The model under review builds one solid part; all positions refer to its coordinate system, in mm. A direction names the side the tool comes from. Coordinates: 2 decimals unless noted, no trailing zeros. Order: outer loops, then holes, each group sorted by start corner. A loop starts at its lowest first (then second) coordinate and runs counter-clockwise, first axis right, second up.
```python
from build123d import *

# Parameters (mm, degrees)
SKETCH1_W                    = 444
SKETCH1_H                    = 24
BASE_FLANGE1_DEPTH           = 1.214
EDGE_FLANGE1_STRIP_W         = 7.284
EDGE_FLANGE1_STRIP_H         = 1.214
EDGE_FLANGE1_STRIP_CUT_DEPTH = 444
EDGE_FLANGE1_DEPTH           = 444
SKETCH9_R                    = 2.5
CUT_EXTRUDE1_DEPTH           = 10


# Sheet-metal steps are written as plain solids
with BuildPart() as part:
    # Sketch1 → Base-Flange1 (new body)
    with BuildSketch(Plane(origin=(0, 0, 0), x_dir=(1, 0, 0), z_dir=(0, 1, 0))):
        Rectangle(SKETCH1_W, SKETCH1_H)
    extrude(amount=BASE_FLANGE1_DEPTH)

    # Edge-Flange1 strip (across the edge) → Edge-Flange1 strip cut (cut)
    with BuildSketch(Plane(origin=(-222, 1.214, 12), x_dir=(0, 0, -1), z_dir=(1, 0, 0))):
        with Locations((-1.214, -0.607)):
            Rectangle(EDGE_FLANGE1_STRIP_W, EDGE_FLANGE1_STRIP_H)
    extrude(amount=EDGE_FLANGE1_STRIP_CUT_DEPTH, mode=Mode.SUBTRACT)

    # Edge-Flange1 section (across the edge) → Edge-Flange1 (add)
    with BuildSketch(Plane(origin=(-222, 1.214, 12), x_dir=(0, 0, -1), z_dir=(1, 0, 0))):
        with BuildLine():
            Line((0, 1.214), (0, 13.786))
            Line((0, 13.786), (1.214, 13.786))
            Line((1.214, 13.786), (1.214, 1.214))
            ThreePointArc((1.214, 1.214), (1.569572368, 0.355572368), (2.428, 0))
            Line((2.428, 0), (2.428, -1.214))
            ThreePointArc((2.428, -1.214), (0.711144735, -0.502855265), (0, 1.214))
        make_face()
    extrude(amount=EDGE_FLANGE1_DEPTH)

    # Sketch9 → Cut-Extrude1 (cut)
    with BuildSketch(Plane.XY.offset(12)):
        with Locations((217, 9.928)):
            Circle(SKETCH9_R)
        with Locations((-217, 9.928)):
            Circle(SKETCH9_R)
    extrude(amount=-CUT_EXTRUDE1_DEPTH, mode=Mode.SUBTRACT)


solid = part.part
```
(1) Machinability: for faces 1 (the face through (-3, 1.214, -1)), 2 (the face through (222, 1, 3)), which of the approach directions +Z, -Z, +X, -X, +Y, -Y give a long, thin tool a straight path to every point of the face, cutting with its end or side? Answer none if there is none.
A:
face 1: -Z, +X, -X, +Y
face 2: +Z, -Z, +X, +Y, -Y
(2) We need section A-A, the plane x = -30. Write out the cut boundary in (y, z), and give its area (3 significant figures).
A:
outline: (0, -12) - (1.21, -12) - (1.21, 9.57) arc R1.21 cw to (2.43, 10.79) - (15, 10.79) - (15, 12) - (2.43, 12) arc R2.43 ccw to (0, 9.57) - close
area: 44.9 mm2
(3) Wall thickness on probe 1 along Y at (x, z) = (-65, -8); probe 2 along Z at (x, y) = (-192, 6.25); probe 3 along Y at (x, z) = (217, 11.3): over which ranges is each line inside the solid? List them lowest first.
A:
probe 1: y = 0 to 1.21
probe 2: z = 10.79 to 12
probe 3: y = 0.72 to 7.43, 12.43 to 15
(4) For pin 1 Ø2 at (x, y) = (-65, 3.5) entering from -Z; pin 2 Ø8 at (x, z) = (149.5, -3) entering from +Y, all flat-tipped, find the tip position at first contact; note any pin that passes through.
A:
pin 1: stops at z = 10.79
pin 2: stops at y = 1.21
(5) We need section B-B, the plane z = 4.5. Write out the cut boundary in (x, y).
A:
outline: (-222, 0) - (222, 0) - (222, 1.21) - (-222, 1.21) - close
